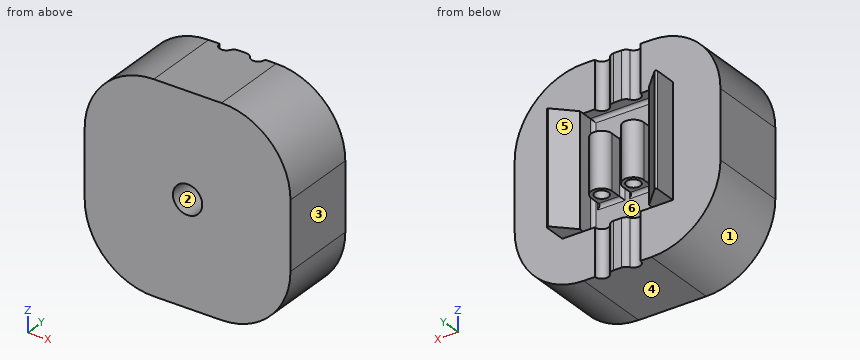
```python
from build123d import *

# Parameters (mm, degrees)
SKETCH2_W               = 29.8
SKETCH2_H               = 29.8
BOSS_EXTRUDE1_DEPTH     = 6.35
SKETCH3_W               = 29.8
SKETCH3_H               = 29.8
BOSS_EXTRUDE2_DEPTH     = 5
FILLET1_R               = 10
SKETCH5_W               = 10
SKETCH5_H               = 16.2
CUT_EXTRUDE1_DEPTH      = 2
SKETCH4_W               = 1.5
SKETCH4_H               = 7.9
SKETCH4_4_W             = 1.5
SKETCH4_4_H             = 7.9
SKETCH6_W               = 3
SKETCH6_H               = 5
BOSS_EXTRUDE3_DEPTH     = 7.9
FILLET3_R               = 0.5
CUT_EXTRUDE2_DEPTH      = 28.248027452
CUT_EXTRUDE2_DEPTH_BACK = 28.248027452
SKETCH7_R               = 1
SKETCH8_R               = 2.125
CUT_EXTRUDE3_DEPTH      = 5
SKETCH9_W               = 3
SKETCH9_H               = 16.2
BOSS_EXTRUDE4_DEPTH     = 0.65
BOSS_EXTRUDE5_DEPTH     = 16.2
FILLET4_R               = 0.2
FILLET5_R               = 1


with BuildPart() as part:
    # Sketch2 → Boss-Extrude1 (new body)
    with BuildSketch(Plane(origin=(0, 0, 0), x_dir=(1, 0, 0), z_dir=(0, 1, 0))):
        Rectangle(SKETCH2_W, SKETCH2_H)
    extrude(amount=BOSS_EXTRUDE1_DEPTH)

    # Sketch3 → Boss-Extrude2 (add)
    with BuildSketch(Plane(origin=(0, 6.35, 0), x_dir=(1, 0, 0), z_dir=(0, 1, 0))):
        Rectangle(SKETCH3_W, SKETCH3_H)
    extrude(amount=BOSS_EXTRUDE2_DEPTH)

    # Fillet1
    fillet1_edges = [part.edges().sort_by_distance(p)[0] for p in [
        (-14.9, 5.675, -14.9),
        (14.9, 5.675, -14.9),
        (14.9, 5.675, 14.9),
        (-14.9, 5.675, 14.9),
    ]]
    fillet(fillet1_edges, radius=FILLET1_R)

    # Sketch5 → Cut-Extrude1 (cut)
    with BuildSketch(Plane(origin=(0, 11.35, 0), x_dir=(1, 0, 0), z_dir=(0, 1, 0))):
        Rectangle(SKETCH5_W, SKETCH5_H)
    extrude(amount=-CUT_EXTRUDE1_DEPTH, mode=Mode.SUBTRACT)



with BuildPart() as body_2:
    # Sketch4 → Revolve1 (revolve)
    with BuildSketch(Plane(origin=(0, 11.35, 0), x_dir=(1, 0, 0), z_dir=(0, 1, 0))):
        with Locations((-3.05, 0)):
            Rectangle(SKETCH4_W, SKETCH4_H)
    revolve(axis=Axis((-2.3, 11.35, -3.95), (0, 0, 1)))


with BuildPart() as body_3:
    # Sketch4<4> → Revolve2 (revolve)
    with BuildSketch(Plane(origin=(0, 11.35, 0), x_dir=(1, 0, 0), z_dir=(0, 1, 0)), mode=Mode.PRIVATE) as revolve2_sk:
        with Locations((3.05, 0)):
            Rectangle(SKETCH4_4_W, SKETCH4_4_H)
    revolve(revolve2_sk.sketch.rotate(Axis((2.3, 11.35, -3.95), (0, 0, 1)), 180), axis=Axis((2.3, 11.35, -3.95), (0, 0, 1)))


with BuildPart() as part_1:
    add(part.part)

    add(body_2.part)  # Boss-Extrude3 merges body 2

    add(body_3.part)  # Boss-Extrude3 merges body 3
    # Sketch6 → Boss-Extrude3 (add)
    with BuildSketch(Plane.XY.offset(3.95)):
        with BuildLine():
            ThreePointArc((-0.8, 11.35), (-2.3, 9.85), (-3.8, 11.35))
            Line((-3.8, 11.35), (-3.8, 6.35))
            Line((-3.8, 6.35), (-0.8, 6.35))
            Line((-0.8, 6.35), (-0.8, 11.35))
        make_face()
        with Locations((2.3, 8.85)):
            Rectangle(SKETCH6_W, SKETCH6_H)
        with BuildLine():
            ThreePointArc((-0.8, 11.35), (-2.3, 12.85), (-3.8, 11.35))
            Line((-3.8, 11.35), (-0.8, 11.35))
        make_face()
        with BuildLine():
            Line((-0.8, 11.35), (-3.8, 11.35))
            ThreePointArc((-3.8, 11.35), (-2.3, 9.85), (-0.8, 11.35))
        make_face()
    extrude(amount=-BOSS_EXTRUDE3_DEPTH)

    # Fillet3
    fillet3_edges = [part_1.edges().sort_by_distance(p)[0] for p in [
        (-0.8, 9.35, 0),
        (-3.8, 9.35, 0),
        (-2.3, 9.35, 3.95),
        (-2.3, 9.35, -3.95),
        (5, 9.35, 0),
        (0, 9.35, -8.1),
        (-5, 9.35, 0),
        (0, 9.35, 8.1),
        (2.3, 9.35, -3.95),
        (0.8, 9.35, 0),
        (3.8, 9.35, 0),
        (2.3, 9.35, 3.95),
    ]]
    fillet(fillet3_edges, radius=FILLET3_R)

    # Sketch7 → Cut-Extrude2 (cut, two sides: drawn at the far end of the back side and taken through both)
    with BuildSketch(Plane.XY.offset(3.95).offset(-CUT_EXTRUDE2_DEPTH_BACK)):
        with Locations((2.3, 11.35)):
            Circle(SKETCH7_R)
        with Locations((-2.3, 11.35)):
            Circle(SKETCH7_R)
    extrude(amount=CUT_EXTRUDE2_DEPTH + CUT_EXTRUDE2_DEPTH_BACK, mode=Mode.SUBTRACT)

    # Sketch8 → Cut-Extrude3 (cut)
    with BuildSketch(Plane.XZ):
        with Locations(Location((0, 0, 0), (0, 0, 270))):
            Circle(SKETCH8_R)
    extrude(amount=-CUT_EXTRUDE3_DEPTH, mode=Mode.SUBTRACT)

    # Sketch9 → Boss-Extrude4 (add)
    with BuildSketch(Plane(origin=(0, 11.35, 0), x_dir=(1, 0, 0), z_dir=(0, 1, 0))):
        with Locations((-6.5, 0)):
            Rectangle(SKETCH9_W, SKETCH9_H)
        with Locations((6.5, 0)):
            Rectangle(SKETCH9_W, SKETCH9_H)
    extrude(amount=BOSS_EXTRUDE4_DEPTH)

    # Sketch10 → Boss-Extrude5 (add)
    with BuildSketch(Plane.XY.offset(8.1)):
        Polygon((8, 15), (8, 12), (5, 12), align=None)
        Polygon((-5, 12), (-8, 15), (-8, 12), align=None)
    extrude(amount=-BOSS_EXTRUDE5_DEPTH)

    # Fillet4
    fillet4_edges = [part_1.edges().sort_by_distance(p)[0] for p in [
        (8, 15, 0),
        (-8, 15, 0),
    ]]
    fillet(fillet4_edges, radius=FILLET4_R)

    # Fillet5
    fillet5_edges = [part_1.edges().sort_by_distance(p)[0] for p in [
        (1.3, 11.35, 11.5),
        (1.3, 11.35, -11.5),
        (-1.3, 11.35, 11.5),
        (-1.3, 11.35, -11.5),
    ]]
    fillet(fillet5_edges, radius=FILLET5_R)


solid = part_1.part
```
Work out the finished part from the listing and answer in its coordinate system (mm). Face numbers are marked on the shaded views. A direction names the side the tool comes from. Round coordinates to 2 decimals unless told otherwise and drop trailing zeros. Write each loop counter-clockwise with the first axis right and the second up, starting at its lowest first coordinate (ties: lowest second). Pieces come first, ordered by that corner, then holes.
1) A cutting plane is placed at B-B on y = 1.75. Determine the outline of the cut face in (x, z) (3 decimals).
2) Determine the mould class of the marked faces 1, 2 and 3 for opening direction Z: pulls with the +Z half, pulls with the -Z half, needs draft (parallel to the pull), parting line crosses it, or undercut.
3) Which of the six approach directions +Z, -Z, +X, -X, +Y, -Y give full straight-line access (tool end or side, diameter ignored) to the marked faces 4, 5 and 6?
4) Consider probe 1 along Y at (x, z) = (2.3, 0.75); probe 2 along X at (y, z) = (2.75, 0) (3 decimals); probe 3 along Y at (x, z) = (0, 0.5). Determine where each line is inside the solid, lowest interval first.
5) A cutting plane is placed at C-C on x = 5.5. Determine the outline of the cut face in (y, z).
6) A cutting plane is placed at A-A on z = 0. Give the number of separate pieces and of enclosed holes in the cut face, and give its area (3 significant figures).
7) Flat-ended cylindrical pins translate along their axes: P1, Ø3.5, axis at x = -6, y = 13.5, coming from the +Z side; P2, Ø1.5, axis at x = -9.5, y = 4, coming from the -Z side; P3, Ø1.6, axis at y = 13.5, z = -3.5, coming from the -X side. Find the tip coordinate at first contact, or state that the pin passes through.
8) A cutting plane is placed at D-D on y = 7.25. Determine the outline of the cut face in (x, z), and give its area (3 significant figures).
Entries:
1. outline: (-14.9, -4.9) arc R10 ccw to (-4.9, -14.9) - (4.9, -14.9) arc R10 ccw to (14.9, -4.9) - (14.9, 4.9) arc R10 ccw to (4.9, 14.9) - (-4.9, 14.9) arc R10 ccw to (-14.9, 4.9) - close; hole circle Ø4.25 at (0, 0)
2. face 1: pulls with the -Z half
2. face 2: undercut
2. face 3: needs draft
3. face 4: -Z, +X, -X, +Y, -Y
3. face 5: +Z, -Z, +Y
3. face 6: +Y
4. probe 1: y = 0 to 10.35, 12.35 to 12.85
4. probe 2: x = -14.9 to -2.125, 2.125 to 14.9
4. probe 3: y = 5 to 9.35
5. outline: (0, -14.88) - (11.35, -14.88) - (11.35, -8.1) - (12.5, -8.1) - (12.5, 8.1) - (11.35, 8.1) - (11.35, 14.88) - (0, 14.88) - close
6. separate pieces: 1
6. enclosed holes: 2
6. area: 323 mm2
7. P1: stops at z = 8.1
7. P2: stops at z = -14.13
7. P3: stops at x = -8
8. outline: (-14.9, -4.9) arc R10 ccw to (-4.9, -14.9) - (4.9, -14.9) arc R10 ccw to (14.9, -4.9) - (14.9, 4.9) arc R10 ccw to (4.9, 14.9) - (-4.9, 14.9) arc R10 ccw to (-14.9, 4.9) - close
8. area: 802 mm2
